Design review of the part built by this model. Coordinates are the model's own, in mm. Round coordinates to 2 decimals unless told otherwise and drop trailing zeros. Order: outer loops, then holes, each group sorted by start corner. A loop starts at its lowest first (then second) coordinate and runs counter-clockwise, first axis right, second up.
Autodesk Inventor part; units mm, degrees
ref_plane "YZ Plane" through (0, 0, 0) normal (1, 0, 0) x (0, 1, 0)
ref_plane "XZ Plane" through (0, 0, 0) normal (0, 1, 0) x (-1, 0, 0)
ref_plane "XY Plane" through (0, 0, 0) normal (0, 0, 1) x (1, 0, 0)
sketch "Sketch1" plane through (0, 0, 0) normal (0, 0, 1) x (1, 0, 0)
  line L0 (-43.2426, 0) -> (42.2071, 0)
  line L1 (0, -15.4497) -> (0, 15.4497)
  line L2 (-25, 10) -> (30, 10)
  line L3 (30, 10) -> (30, -10)
  line L4 (30, -10) -> (-25, -10)
  line L5 (-30, -5) -> (-30, 5)
  arc A0 (-25, 10) -> (-30, 5) centre (-25, 5) ccw
  arc A1 (-30, -5) -> (-25, -10) centre (-25, -5) ccw
  point P0 (0, 0)
  point P1 (-30, 10)
  point P2 (-30, -10)
  dimension "d0" = 60
  dimension "d1" = 20
  dimension "d2" = 30
  dimension "d3" = 10
  dimension "d6" = 5
extrude "Extrusion1" add sketch "Sketch1" along normal blind 2.8
sketch "Sketch2" plane through (0, 0, 2.8) normal (0, 0, 1) x (1, 0, 0)
  line L0 (30, 10) -> (30, -10)
  line L1 (-30, -5) -> (-30, 5)
  circle A0 centre (-26.7, 0) radius 1.5
  circle A1 centre (26.2, 0) radius 1.5
  circle A2 centre (-5.65, 0) radius 1.5
  point P0 (0, 0)
  dimension "d7" = 3
  dimension "d8" = 3
  dimension "d9" = 3.8
  dimension "d10" = 3.3
extrude "Extrusion2" cut sketch "Sketch2" against normal blind 10
equation "\"d2\" = 0.5 * d0"
equation "\"d3\" = 0.5 * d1"
properties part number "Acrylic_PitchServoSupport_2"
1) To check wall thickness, follow line 1 along Y through (x, z) = (26.2, 0.95); line 2 along X through (y, z) = (-1, 0.3); line 3 along X through (y, z) = (0.25, 2). State the ranges of each line that lie inside material, in increasing order.
Results:
line 1: y = -10 to -1.5, 1.5 to 10
line 2: x = -30 to -27.82, -25.58 to -6.77, -4.53 to 25.08, 27.32 to 30
line 3: x = -30 to -28.18, -25.22 to -7.13, -4.17 to 24.72, 27.68 to 30
2) Take a section at C-C on x = 26.2. Give the boundary of the cut face in (y, z), plus the area to 3 significant figures.
Results:
outline: (-10, 0) - (-1.5, 0) - (-1.5, 2.8) - (-10, 2.8) - close; (1.5, 0) - (10, 0) - (10, 2.8) - (1.5, 2.8) - close
area: 47.6 mm2
3) The part is to be moulded in two halves that separate along X. For faces 1 (the face through (-29, 8, 1)), 2 (the face through (2, 10, 1)), 3 (the face through (27.63, 0.45, 1.42)), say which applies: released by +X, released by -X, zero draft, split by the parting line, or undercut.
Results:
face 1: released by -X
face 2: zero draft
face 3: undercut
4) Take a section at D-D on x = -26.7. Give the boundary of the cut face in (y, z).
Results:
outline: (-9.7, 0) - (-1.5, 0) - (-1.5, 2.8) - (-9.7, 2.8) - close; (1.5, 0) - (9.7, 0) - (9.7, 2.8) - (1.5, 2.8) - close
5) Take a section at B-B on z = 1.8. Give the boundary of the cut face in (x, y).
Results:
outline: (-30, -5) arc R5 ccw to (-25, -10) - (30, -10) - (30, 10) - (-25, 10) arc R5 ccw to (-30, 5) - close; hole circle Ø3 at (-26.7, 0); hole circle Ø3 at (-5.65, 0); hole circle Ø3 at (26.2, 0)
6) Take a section at A-A on y = 0. Give the boundary of the cut face in (x, z), plus the area to 3 significant figures.
Results:
outline: (-30, 0) - (-28.2, 0) - (-28.2, 2.8) - (-30, 2.8) - close; (-25.2, 0) - (-7.15, 0) - (-7.15, 2.8) - (-25.2, 2.8) - close; (-4.15, 0) - (24.7, 0) - (24.7, 2.8) - (-4.15, 2.8) - close; (27.7, 0) - (30, 0) - (30, 2.8) - (27.7, 2.8) - close
area: 143 mm2
7) Clearance check with a flat-ended pin moving along its axis: P1, Ø1.8, axis at x = -5.65, y = 0, coming from the +Z side. State where the tip first meets the part, or that it passes through.
Results:
P1: passes through
